Here's how the part is built. I have some questions about the finished solid (model axes, mm). Face numbers are marked on the shaded views. Coordinates: 2 decimals unless noted, no trailing zeros. Write each question's results on one line, items separated by ' | '. Start each with the question number.
from build123d import *

# Parameters (mm, degrees)
CONG_1_R          = 1
D_GAGEMENT_M121_D = 13.5
CHANFREIN1_SIZE   = 0.5


with BuildPart() as part:
    # Lissage1: read off the stored shape, not the designer's step
    # Lissage1: loft between two sections, ruled curve by curve
    lissage1_from = [
        Edge.make_bspline([(-10.806835439, 13, -7.225808453), (3.644781468, 13, -28.83947933), (25.258452345, 13, -14.387862424), (10.806835439, 13, 7.225808453), (-3.644781468, 13, 28.83947933), (-25.258452345, 13, 14.387862424), (-10.806835439, 13, -7.225808453)], [0, 0, 0, 0, 0.5, 0.5, 0.5, 1, 1, 1, 1], 3, [1, 0.333333333, 0.333333333, 1, 0.333333333, 0.333333333, 1]),
    ]
    lissage1_to = [
        Edge.make_bspline([(-6.654259826, 0, -8.759042537), (10.863825248, 0, -22.06756219), (24.1723449, 0, -4.549477116), (6.654259826, 0, 8.759042537), (-10.863825248, 0, 22.06756219), (-24.1723449, 0, 4.549477116), (-6.654259826, 0, -8.759042537)], [0, 0, 0, 0, 0.5, 0.5, 0.5, 1, 1, 1, 1], 3, [1, 0.333333333, 0.333333333, 1, 0.333333333, 0.333333333, 1]),
    ]
    lissage1 = Solid(Shell([*[Face.make_surface_from_curves(lissage1_from[k], lissage1_to[k]) for k in range(1)], Face(Wire(lissage1_from)), Face(Wire(lissage1_to))]))
    add(lissage1)

    # Congé1
    cong_1_edges = [part.edges().sort_by_distance(p)[0] for p in [
        (6.654259826, 0, 8.759042537),
    ]]
    fillet(cong_1_edges, radius=CONG_1_R)

    # Dégagement M121 (through all)
    with Locations(Plane(origin=(0, 13, 0), x_dir=(1, 0, 0), z_dir=(0, 1, 0))):
        with Locations((0, 0)):
            Hole(D_GAGEMENT_M121_D / 2)

    # Chanfrein1
    chanfrein1_edges = [part.edges().sort_by_distance(p)[0] for p in [
        (6.75, 0, 0),
    ]]
    chamfer(chanfrein1_edges, length=CHANFREIN1_SIZE)


solid = part.part
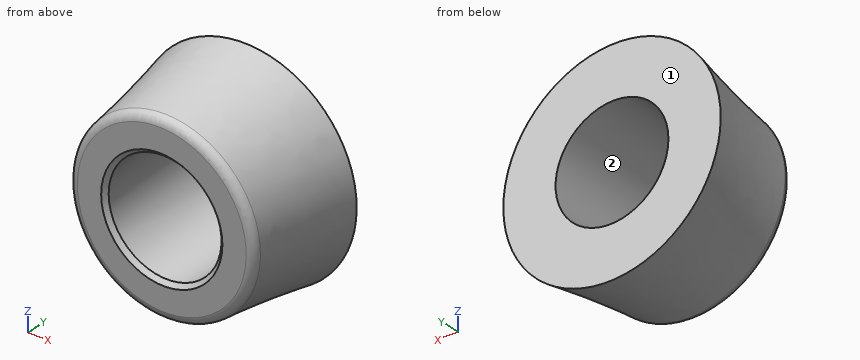
1) For pin 1 Ø1.5 at (x, y) = (-5.5, 5.5) entering from +Z; pin 2 Ø2 at (x, y) = (0.5, 6) entering from +Z; pin 3 Ø12 at (x, z) = (0, 0) entering from +Y; pin 4 Ø1 at (y, z) = (8.5, -5) entering from +X, each with a flat end and sliding along its axis, tell me the tip position at first contact or that it passes through.
2) Please list where these lines run through material, in increasing order: line 1 (X direction, y = 1.75, z = -2.5); line 2 (Z direction, x = 0, y = 10); line 3 (X direction, y = 4.5, z = 0). Write a range as [from, to].
3) We'd pull the mould along X, two halves only. Please class the marked faces 1 and 2: pulls with the +X half, pulls with the -X half, needs draft (parallel to the pull), parting line crosses it, or undercut.
Output:
1) pin 1: stops at z = 10.7 | pin 2: stops at z = 11.91 | pin 3: passes through | pin 4: stops at x = 11.32
2) line 1: x = [-10.91, -6.27], [6.27, 10.91] | line 2: z = [-12.43, -6.75], [6.75, 12.43] | line 3: x = [-11.54, -6.75], [6.75, 11.54]
3) face 1: needs draft | face 2: undercut
